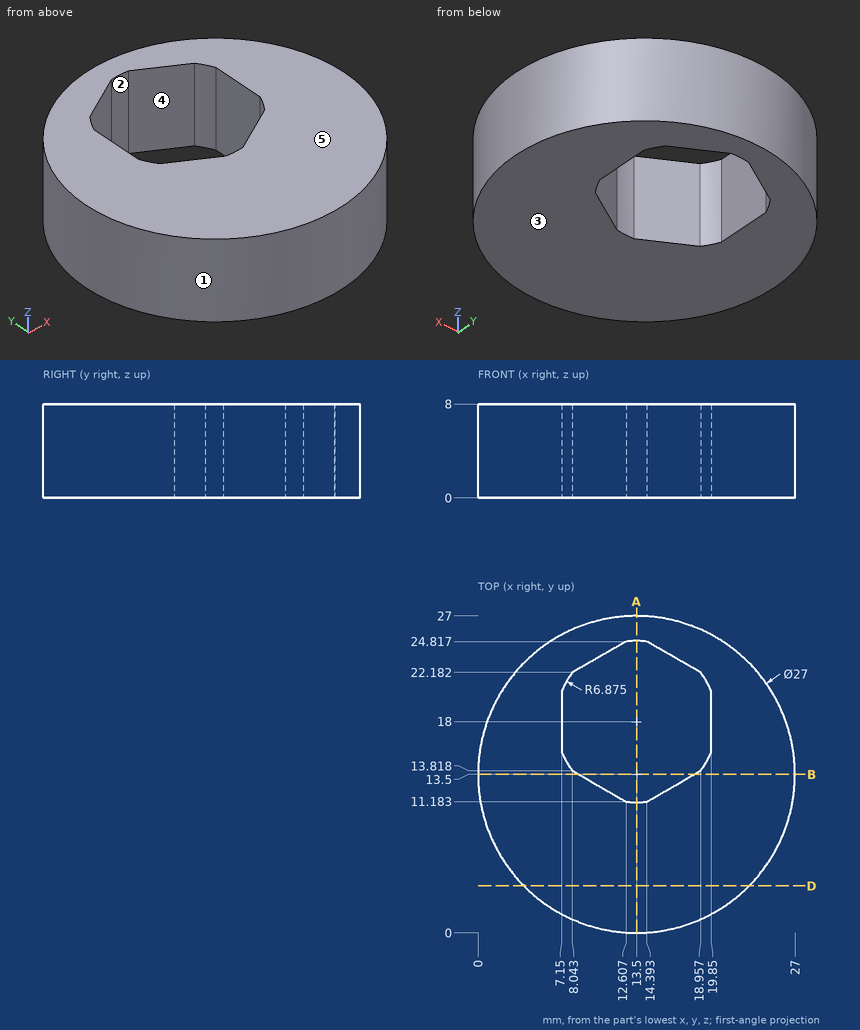
Part print with two shaded views. Sizes in mm from the minimum x, y, z corner. A direction names the side the tool comes from. Coordinates: 2 decimals unless noted, no trailing zeros. Write each loop counter-clockwise with the first axis right and the second up, starting at its lowest first coordinate (ties: lowest second). Pieces come first, ordered by that corner, then holes.
(1) Cut at A-A on x = 13.5. List the corners of the cut face in (y, z) (1 decimal), and give its area (3 significant figures).
(2) Drill centre lines: line 1 (Y direction, x = 13.75, z = 5.5); line 2 (Y direction, x = 11.5, z = 7); line 3 (X direction, y = 18.75, z = 1.75). Where is each one in solid material? Low to high.
(3) Mould opens along Y. For the marked faces 1, 2 and 3 say: pulls with the +Y half, pulls with the -Y half, needs draft (parallel to the pull), parting line crosses it, or undercut.
(4) Pin check, flat tips, straight feed: pin 1 Ø1 at (x, z) = (8.5, 7) entering from +Y; pin 2 Ø4 at (y, z) = (19, 4.5) entering from -X; pin 3 Ø1 at (y, z) = (16, 5.5) entering from -X; pin 4 Ø8 at (x, y) = (19, 22) entering from -Z. Stop position of each tip, or through.
(5) 3-axis set-ups, long thin cutter, end or side, ignore diameter. For the marked faces 4 and 5: which of +Z, -Z, +X, -X, +Y, -Y reach the whole face in a straight line?
(6) Cut at D-D on y = 4. List the corners of the cut face in (x, z), and give its area (3 significant figures).
(7) Cut at B-B on y = 13.5. List the corners of the cut face in (x, z), and give its area (4 significant figures).
Working result:
1. outline: (0, 0) - (11.1, 0) - (11.1, 8) - (0, 8) - close; (24.9, 0) - (27, 0) - (27, 8) - (24.9, 8) - close
1. area: 106 mm2
2. line 1: y = 0 to 11.13, 24.87 to 27
2. line 2: y = 0.15 to 11.82, 24.18 to 26.85
2. line 3: x = 1.06 to 7.15, 19.85 to 25.94
3. face 1: parting line crosses it
3. face 2: undercut
3. face 3: needs draft
4. pin 1: stops at y = 26.23
4. pin 2: stops at x = 0.46
4. pin 3: stops at x = 0.15
4. pin 4: stops at z = 0
5. face 4: +Z, -Z
5. face 5: +Z, +X, -X, +Y, -Y
6. outline: (3.91, 0) - (23.09, 0) - (23.09, 8) - (3.91, 8) - close
6. area: 153 mm2
7. outline: (0, 0) - (8.59, 0) - (8.59, 8) - (0, 8) - close; (18.41, 0) - (27, 0) - (27, 8) - (18.41, 8) - close
7. area: 137.5 mm2
